Autodesk Inventor part; units mm, degrees
ref_plane "YZ Plane" through (0, 0, 0) normal (1, 0, 0) x (0, 1, 0)
ref_plane "XZ Plane" through (0, 0, 0) normal (0, 1, 0) x (-1, 0, 0)
ref_plane "XY Plane" through (0, 0, 0) normal (0, 0, 1) x (1, 0, 0)
sketch "Sketch1" plane through (0, 0, 0) normal (0, 1, 0) x (-1, 0, 0)
  line L0 (0, 0) -> (38.1, 0)
  line L1 (38.1, 0) -> (38.1, -201.295)
  line L2 (38.1, -201.295) -> (0, -201.295)
  line L3 (0, -201.295) -> (0, 0)
  dimension "d0" = 201.295
  dimension "d1" = 38.1
extrude "Extrusion1" add sketch "Sketch1" along normal blind 2.54
sketch "Sketch2" plane through (0, 2.54, 0) normal (0, 1, 0) x (1, 0, 0)
  line L0 (-38.1, 201.295) -> (-38.1, 0)
  line L1 (-38.1, 0) -> (0, 0)
  line L2 (0, 0) -> (0, 201.295)
  line L3 (-38.1, 0) -> (0, 0)
  line L4 (0, 0) -> (0, 2.535)
  line L5 (0, 2.535) -> (-38.1, 2.535)
  line L6 (-38.1, 2.535) -> (-38.1, 0)
  line L7 (0, 201.295) -> (-38.1, 201.295)
  line L8 (-38.1, 201.295) -> (-38.1, 198.7847)
  line L9 (-38.1, 198.7847) -> (0, 198.7847)
  line L10 (0, 198.7847) -> (0, 201.295)
extrude "Extrusion2" add sketch "Sketch2" along normal blind 38.1 contours L7 L2 L9 L0 | L5 L2 L1 L0
sketch "Sketch3" plane through (0, 0, -201.295) normal (0, 0, -1) x (-1, 0, 0)
  line L0 (38.1, 40.64) -> (0, 40.64)
  line L1 (19.05, 40.64) -> (19.05, 0)
  line L2 (38.1, 0) -> (0, 0)
  line L3 (0, 0) -> (0, 40.64)
  line L4 (0, 20.32) -> (38.1, 20.32)
  line L5 (38.1, 2.54) -> (38.1, 40.64)
  circle A0 centre (19.05, 35.9001) radius 13.4747
  circle A1 centre (32.5247, 35.9001) radius 1.7907
  circle A2 centre (5.5753, 35.9001) radius 1.7907
  dimension "d11" = 26.9494
  dimension "d12" = 3.5814
  dimension "d13" = 3.5814
extrude "Extrusion3" cut sketch "Sketch3" against normal blind 246.0625 contours A1 A0 | A0 A1 | A2 A0 | A0 A2
properties part number "LiftBrace"
Geometry: final body of the model. Coordinates: model frame, mm. A direction names the side the tool comes from. Round coordinates to 2 decimals unless told otherwise and drop trailing zeros. Order: outer loops, then holes, each group sorted by start corner. A loop starts at its lowest first (then second) coordinate and runs counter-clockwise, first axis right, second up. Notation, with made-up numbers: M 76.5,13 L 106.5,13 A7 ccw 106.5,26 Z; hole C 55,-7 d4. An arc over 180 degrees is marked long. Use one line per item in the form item = value. Start each with the question number.
Q1. Pin query (flat end, axial travel): pin 1 Ø4 at (x, y) = (-32.52, 35.9) entering from +Z; pin 2 Ø6 at (x, z) = (-4, -149) entering from +Y. Return the tip coordinate at first contact, or that it passes through.
Q2. Material intervals for line 1 (Z direction, x = -19, y = 22) (3 decimals); line 2 (Y direction, x = -25, z = -25.5), sorted ascending. Write a range as [from, to].
Q3. Cut plane A-A (y = 14). Return loops of the section in (x, z) (3 decimals), and give its area (3 significant figures).
Q4. Cut plane C-C (z = -128.5). Return loops of the section in (x, y).
Q5. Access query for faces 1 (the face through (-19, 2.54, -99)), 2 (the face through (-19, 0, -99)). Directions: +Z, -Z, +X, -X, +Y, -Y. A direction counts if a zero-diameter tool reaches every point of the face in a straight line with its end or side. Return the directions, or none.
Q6. Mould query, pull axis X, two halves, no side actions, for faces 3 (the face through (-19, 21, -198.785)), 4 (the face through (0, 1, -101)), 5 (the face through (-38.1, 1, -100)), 6 (the face through (-6.54, 37.41, -200.06)). Classes: +X half, -X half, draft (parallel to the pull), parting line (faces both ways), or undercut.
Q7. Cut plane B-B (x = -17). Return loops of the section in (y, z) (3 decimals), and give its area (3 significant figures).
Geometry results:
q1.pin_1 = 0
q1.pin_2 = 2.54
q2.line_1 = [-201.295, -198.785], [-2.535, 0]
q2.line_2 = [0, 2.54]
q3.outline = M -38.1,-201.295 L 0,-201.295 L 0,-198.785 L -38.1,-198.785 Z; M -38.1,-2.535 L 0,-2.535 L 0,0 L -38.1,0 Z
q3.area = 192 mm^2
q4.outline = M -38.1,0 L 0,0 L 0,2.54 L -38.1,2.54 Z
q5.face_1 = +X, -X, +Y
q5.face_2 = +Z, -Z, +X, -X, -Y
q6.face_3 = draft
q6.face_4 = +X half
q6.face_5 = -X half
q6.face_6 = undercut
q7.outline = M 0,-201.295 L 40.64,-201.295 L 40.64,-198.785 L 2.54,-198.785 L 2.54,-2.535 L 40.64,-2.535 L 40.64,0 L 0,0 Z
q7.area = 704 mm^2
